Check sheet for the drawn part. Datum: minimum x, y, z corner. Units: mm. Give positions to 0.01 mm unless a question says otherwise; leave off trailing zeros. Order: outer loops, then holes, each group sorted by start corner. A loop starts at its lowest first (then second) coordinate and runs counter-clockwise, first axis right, second up.
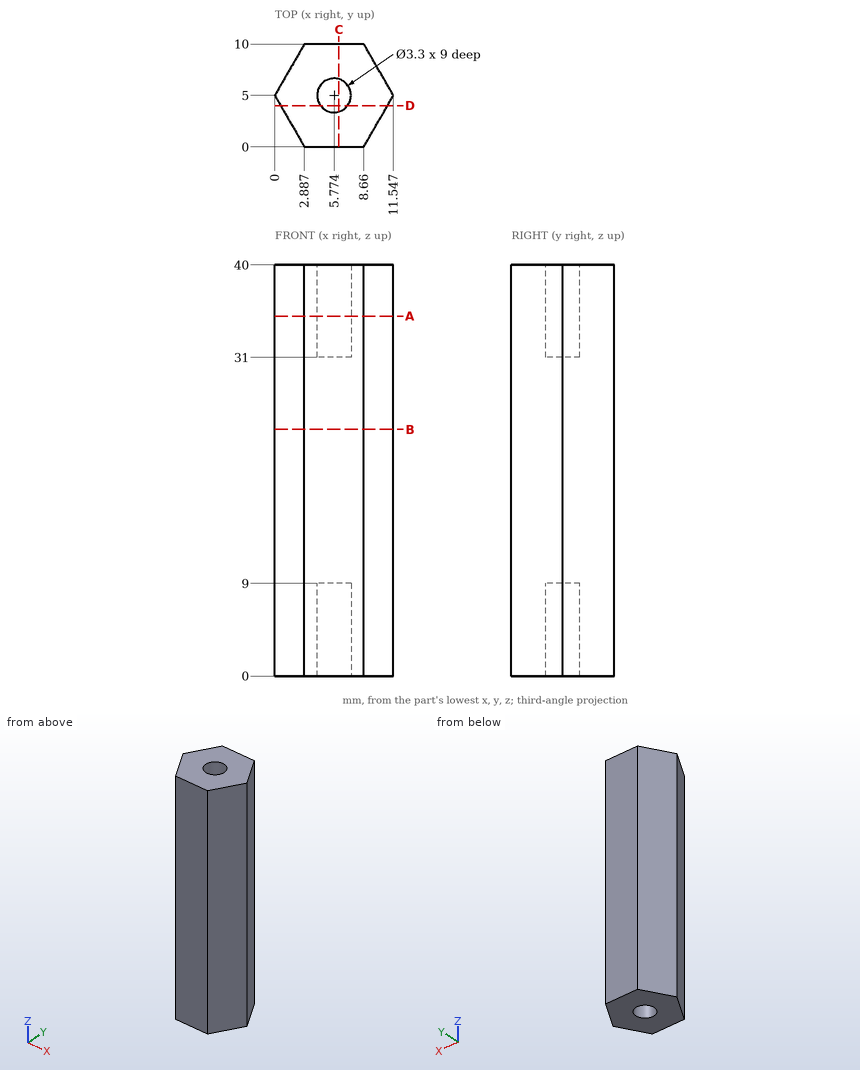
Q1. Sectioned sample at A-A, the plane z = 35. Record the cut outline in (x, y).
Q2. Sectioned sample at D-D, the plane y = 4. Record the cut outline in (x, z) (1 decimal).
Q3. Sectioned sample at C-C, the plane x = 6.25. Record the cut outline in (y, z).
Q4. Sectioned sample at B-B, the plane z = 24. Record the cut outline in (x, y).
Q5. Go/stop test with flat-tipped pins: P1, Ø4, axis at y = 6, z = 25, coming from the -X side; P2, Ø2.5, axis at x = 5.77, y = 5, coming from the +Z side; P3, Ø2.5, axis at x = 6, y = 5, coming from the -Z side. Record where each tip stops, or that it passes through.
Q6. Material ranges on line 1 (X direction, y = 3.5, z = 34) (1 decimal); line 2 (Y direction, x = 4.5, z = 33); line 3 (Y direction, x = 6, z = 3) (1 decimal), recorded low to high.
Filled in:
1. outline: (0, 5) - (2.89, 0) - (8.66, 0) - (11.55, 5) - (8.66, 10) - (2.89, 10) - close; hole circle Ø3.3 at (5.77, 5)
2. outline: (0.6, 0) - (4.5, 0) - (4.5, 9) - (7.1, 9) - (7.1, 0) - (11, 0) - (11, 40) - (7.1, 40) - (7.1, 31) - (4.5, 31) - (4.5, 40) - (0.6, 40) - close
3. outline: (0, 0) - (3.42, 0) - (3.42, 9) - (6.58, 9) - (6.58, 0) - (10, 0) - (10, 40) - (6.58, 40) - (6.58, 31) - (3.42, 31) - (3.42, 40) - (0, 40) - close
4. outline: (0, 5) - (2.89, 0) - (8.66, 0) - (11.55, 5) - (8.66, 10) - (2.89, 10) - close
5. P1: stops at x = 0
5. P2: stops at z = 31
5. P3: stops at z = 9
6. line 1: x = 0.9 to 5.1, 6.5 to 10.7
6. line 2: y = 0 to 3.95, 6.05 to 10
6. line 3: y = 0 to 3.4, 6.6 to 10
